Source: CAD feature listing. Evaluate the final solid. Frame: model axes, mm. Give positions to 0.01 mm unless a question says otherwise; leave off trailing zeros. Order: outer loops, then holes, each group sorted by start corner. A loop starts at its lowest first (then second) coordinate and runs counter-clockwise, first axis right, second up. Notation, with made-up numbers: M 72.5,81 L 93.5,81 A37 ccw 93.5,119 Z; hole C 42.5,61.25 d1. An arc over 180 degrees is marked long. Use CSV: the item, a comma, the result in double quotes. Start each with the question number.
Item 1: Section query C-C on x = 376. Return loops of the section in (y, z) (3 decimals), and give its area (3 significant figures).
Item 2: Ray query, probe 1 along Y at (x, z) = (215.9, 0.95) (3 decimals); probe 2 along X at (y, z) = (47, 1.45); probe 3 along X at (y, z) = (322.5, 2.3). Return the intervals inside material, ascending. Write a range as from..to.
Item 3: Section query A-A on z = 1. Count the separate pieces of the cut face and the enclosed holes in it, and give its area (3 significant figures).
Item 4: Section query B-B on y = 396. Return loops of the section in (x, z) (1 decimal).
Item 5: First-contact query: pin 1 (12 mm diameter, centred on x = 209, y = 422, fed in from -Z); pin 2 (1.6 mm diameter, centred on x = 430.5, z = 1.5, fed in from -Y) (3 decimals); pin 3 (1 mm diameter, centred on x = 210, z = 3, fed in from +Y) (3 decimals); pin 4 (1.6 mm diameter, centred on x = 215.5, z = 2, fed in from +Y) (3 decimals). Flat tips, straight axial feed; report the tip coordinate or a pass-through.
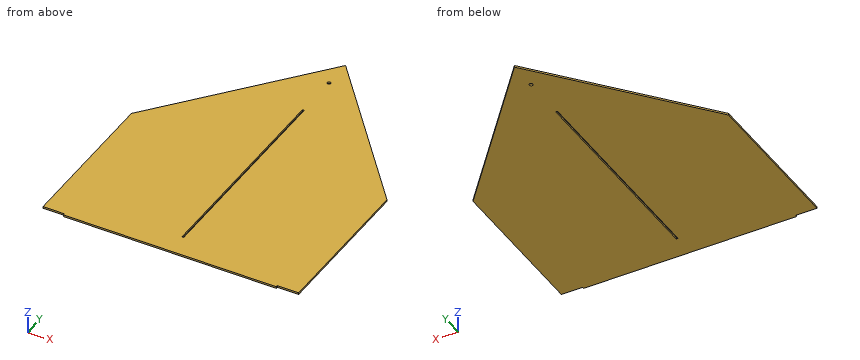
Autodesk Inventor part; units mm, degrees
ref_plane "YZ Plane" through (0, 0, 0) normal (1, 0, 0) x (0, 1, 0)
ref_plane "XZ Plane" through (0, 0, 0) normal (0, 1, 0) x (-1, 0, 0)
ref_plane "XY Plane" through (0, 0, 0) normal (0, 0, 1) x (1, 0, 0)
sketch "Sketch1" plane through (0, 0, 0) normal (0, 0, 1) x (1, 0, 0)
  line L0 (0, 0) -> (-3.175, 0)
  line L1 (-3.175, 0) -> (-3.175, 381)
  line L2 (-3.175, 381) -> (0, 381)
  line L3 (0, 381) -> (0, 0)
  line L4 (-3.175, -38.1) -> (-555.625, -38.1)
  line L5 (-555.625, -38.1) -> (-555.625, 419.1)
  line L6 (-555.625, 419.1) -> (-3.175, 419.1)
  line L7 (-3.175, 419.1) -> (-3.175, -38.1)
  line L8 (-555.625, 190.5) -> (-282.575, -38.1)
  line L9 (-555.625, 190.5) -> (-282.575, 419.1)
  circle A0 centre (-503.174, 190.5) radius 3.175
  line L10 (-41.275, 188.9125) -> (-422.275, 188.9125)
  line L11 (-422.275, 188.9125) -> (-422.275, 192.0875)
  line L12 (-422.275, 192.0875) -> (-41.275, 192.0875)
  line L13 (-41.275, 192.0875) -> (-41.275, 188.9125)
  point P0 (-1.5875, 0)
  point P1 (-3.175, 0)
  point P2 (-3.175, 381)
  point P3 (-41.275, 190.5)
  dimension "d0" = 3.175
  dimension "d1" = 381
  dimension "d2" = 552.45
  dimension "d3" = 457.2
  dimension "d4" = 38.1
  dimension "d5" = 228.6
  dimension "d6" = 279.4
  dimension "d7" = 228.6
  dimension "d9" = 6.35
  dimension "d10" = 228.6
  dimension "d11" = 499.999
  dimension "d12" = 279.4
  dimension "d15" = 381
  dimension "d16" = 3.175
  dimension "d17" = 227.0125
  dimension "d18" = 38.1
extrude "Extrusion1" add sketch "Sketch1" along normal blind 3.175 contours L0 L1 L2 L3 | L7 L4 L8 L9 L6 L1
move or copy body "Move Body1" bodies to move or copy 1 copy no rotation origin (0, 0, 0) rotation axis (0, 0, 1) rotation angle -90
move or copy body "Move Body2" bodies to move or copy 1 copy no translate (25.4, 0, 0)
properties part number "side"
Verdict:
1,outline,"M 0,0 L 364.394,0 L 364.394,3.175 L 0,3.175 Z"
1,area,"1,160 mm2"
2,probe 1,"0..41.275, 422.275..499.999, 506.349..555.625"
2,probe 2,"-12.7..214.31, 217.49..444.5"
2,probe 3,"20.73..214.31, 217.49..411.07"
3,separate pieces,"1"
3,enclosed holes,"2"
3,area,"190,000 mm2"
4,outline,"M 82.3,0 L 214.3,0 L 214.3,3.2 L 82.3,3.2 Z; M 217.5,0 L 349.5,0 L 349.5,3.2 L 217.5,3.2 Z"
5,pin 1,"z = 0"
5,pin 2,"y = 3.175"
5,pin 3,"y = 549.175"
5,pin 4,"y = 555.625"
